For this review, take the finished solid that the model builds, in its own axes (mm). A direction names the side the tool comes from. Give positions to 0.01 mm unless a question says otherwise; leave off trailing zeros. Write each loop counter-clockwise with the first axis right and the second up, starting at its lowest first coordinate (ties: lowest second). Pieces come first, ordered by that corner, then holes. Notation, with made-up numbers: M 84.5,88.25 L 137.5,88.25 A27 cw 137.5,110.25 Z; hole C 20,-19 d8. An arc over 180 degrees is marked long. Use one line per item in the form item = value. Start each with the question number.
Q1. Consider section A-A on y = 0. Write out the cut boundary in (x, z) (3 decimals), and give its area (3 significant figures).
Q2. Clearance check with flat-ended pins moving along their axes: pin 1 Ø1.5 at (x, z) = (-5.5, 9) entering from +Y; pin 2 Ø3 at (y, z) = (3, -4) entering from +X; pin 3 Ø1.4 at (x, z) = (-0.5, -4.5) entering from +Y. State where each tip first meets the part, or that it passes through.
Q3. Tool access review of faces 1 (the flat face through (5.1, 3, -4)), 2 (the flat face through (0, 8.2, 14)), 3 (the flat face through (4.6, 3, -4)): name each direction out of +Z, -Z, +X, -X, +Y, -Y from which nothing blocks a thin tool from reaching the whole face with its end or side.
Q4. For probe 1 along Y at (x, z) = (1.25, -0.5); probe 2 along X at (y, z) = (-3.75, -0.25); probe 3 along Z at (x, y) = (-3.5, -1), list the stretches that pass through material, from the lowest coordinate up. Write a range as [from, to].
Q5. Mouldability with a two-part tool opening along Y and no side actions: class faces 4 (the cylindrical face through (-2.17, 9.76, 14.49)), 5 (the flat face through (0, 5.33, -4)), 6 (the flat face through (0, -5.83, -4)) as released by +Y, released by -Y, zero draft, split by the parting line, or undercut.
Q6. Consider section B-B on x = 0. Write out the cut boundary in (y, z) (3 decimals).
Q7. Consider section C-C on z = 4.5. Write out the cut boundary in (x, y), and give its area (3 significant figures).
Autodesk Inventor part; units mm, degrees
ref_plane "YZ Plane" through (0, 0, 0) normal (1, 0, 0) x (0, 1, 0)
ref_plane "XZ Plane" through (0, 0, 0) normal (0, 1, 0) x (-1, 0, 0)
ref_plane "XY Plane" through (0, 0, 0) normal (0, 0, 1) x (1, 0, 0)
sketch "スケッチ1" plane through (0, 0, 0) normal (0, 0, 1) x (1, 0, 0)
  circle A0 centre (0, 0) radius 8
  dimension "d0" = 16
extrude "押し出し1" add sketch "スケッチ1" along normal blind 14
sketch "スケッチ2" plane through (0, 0, 14) normal (0, 0, 1) x (1, 0, 0)
  circle A0 centre (0, 0) radius 10
  dimension "d3" = 20
extrude "押し出し2" add sketch "スケッチ2" along normal blind 2.5
fillet "フィレット1" radius 1.5 1 edges at (-10, 0, 16.5)
sketch "スケッチ3" plane through (0, 0, 16.5) normal (0, 0, 1) x (1, 0, 0)
  circle A0 centre (0, 0) radius 6.665
  dimension "d7" = 13.33
extrude "押し出し3" add sketch "スケッチ3" along normal blind 2.5
sketch "スケッチ4" plane through (0, 0, 0) normal (0, 0, -1) x (-1, 0, 0)
  line L0 (-1.35, 5.83) -> (1.35, 5.83)
  line L1 (1.35, 5.83) -> (1.35, 5.33)
  line L2 (1.35, 5.33) -> (-1.35, 5.33)
  line L3 (-1.35, 5.33) -> (-1.35, 5.83)
  line L4 (0, -14) -> (0, 14)
  line L5 (14, 0) -> (-14, 0)
  line L6 (-1.35, -5.83) -> (1.35, -5.83)
  line L7 (1.35, -5.83) -> (1.35, -5.33)
  line L8 (1.35, -5.33) -> (-1.35, -5.33)
  line L9 (-1.35, -5.33) -> (-1.35, -5.83)
  line L10 (4.6, 4.36) -> (5.1, 4.36)
  line L11 (5.1, 4.36) -> (5.1, 1.66)
  line L12 (5.1, 1.66) -> (4.6, 1.66)
  line L13 (4.6, 1.66) -> (4.6, 4.36)
  line L14 (4.6, -4.36) -> (5.1, -4.36)
  line L15 (5.1, -4.36) -> (5.1, -1.66)
  line L16 (5.1, -1.66) -> (4.6, -1.66)
  line L17 (4.6, -1.66) -> (4.6, -4.36)
  line L18 (-4.6, 4.36) -> (-5.1, 4.36)
  line L19 (-5.1, 4.36) -> (-5.1, 1.66)
  line L20 (-5.1, 1.66) -> (-4.6, 1.66)
  line L21 (-4.6, 1.66) -> (-4.6, 4.36)
  line L22 (-4.6, -1.66) -> (-4.6, -4.36)
  line L23 (-4.6, -4.36) -> (-5.1, -4.36)
  line L24 (-5.1, -4.36) -> (-5.1, -1.66)
  line L25 (-5.1, -1.66) -> (-4.6, -1.66)
  point P0 (0, 0)
  point P1 (0, 5.83)
  point P2 (0, -5.83)
  dimension "d10" = 2.7
  dimension "d11" = 5.83
  dimension "d12" = 0.5
  dimension "d13" = 2.7
  dimension "d14" = 0.5
  dimension "d15" = 4.36
  dimension "d16" = 5.1
extrude "押し出し4" add sketch "スケッチ4" along normal blind 7.16
chamfer "面取り1" distance 0.5 angle 45 12 edges at (-4.85, -4.36, -7.16) (-4.85, -1.66, -7.16) (-4.85, 1.66, -7.16) (-4.85, 4.36, -7.16) (-1.35, 5.58, -7.16) (1.35, 5.58, -7.16) (4.85, 4.36, -7.16) (4.85, 1.66, -7.16) (4.85, -1.66, -7.16) (4.85, -4.36, -7.16) (1.35, -5.58, -7.16) (-1.35, -5.58, -7.16)
equation "\"d13\" = d10"
equation "\"d14\" = d12"
properties part number "switch"
Working result:
q1.outline = M -10,14 L -8,14 L -8,0 L 8,0 L 8,14 L 10,14 L 10,15 A1.5 ccw 8.5,16.5 L 6.665,16.5 L 6.665,19 L -6.665,19 L -6.665,16.5 L -8.5,16.5 A1.5 ccw -10,15 Z
q1.area = 306 mm²
q2.pin_1 = 6.44
q2.pin_2 = 5.1
q2.pin_3 = 5.83
q3.face_1 = -Z, +X, +Y, -Y
q3.face_2 = -Z
q3.face_3 = -Z, +Y, -Y
q4.probe_1 = [-5.83, -5.33], [5.33, 5.83]
q4.probe_2 = [-5.1, -4.6], [4.6, 5.1]
q4.probe_3 = [0, 19]
q5.face_4 = split by the parting line
q5.face_5 = undercut
q5.face_6 = released by -Y
q6.outline = M -10,14 L -8,14 L -8,0 L -5.83,0 L -5.83,-7.16 L -5.33,-7.16 L -5.33,0 L 5.33,0 L 5.33,-7.16 L 5.83,-7.16 L 5.83,0 L 8,0 L 8,14 L 10,14 L 10,15 A1.5 ccw 8.5,16.5 L 6.665,16.5 L 6.665,19 L -6.665,19 L -6.665,16.5 L -8.5,16.5 A1.5 ccw -10,15 Z
q7.outline = C 0,0 d16
q7.area = 201 mm²
